Here's how the part is built. I have some questions about the finished solid (model axes, mm). Give positions to 0.01 mm unless a question says otherwise; leave off trailing zeros. Order: outer loops, then holes, each group sorted by start corner. A loop starts at its lowest first (then second) coordinate and runs counter-clockwise, first axis right, second up. Notation, with made-up numbers: (40.5, 53.5) - (98.5, 53.5) arc R15 ccw to (98.5, 69.5) - close; hole circle Ø8 at (41.25, 40). An arc over 180 degrees is marked (long way). One line per question, with ' | ' between items.
from build123d import *

# Parameters (mm, degrees)
F1_R     = 12
F2_DEPTH = 15


with BuildPart() as f2:
    # F1 (on face) → F2 (new body)
    with BuildSketch(Plane.XY):
        with BuildLine():
            ThreePointArc((17.8272945993, -129.4724747228), (30.8870152167, -67.4921341785), (35.2682027622, -4.3025455402))
            add(Edge.make_bspline(
                [(35.2682027622, -4.3025455402), (35.2682027622, -2.8630395725), (34.7940906326, 4.5484558025), (29.9290871814, 17.4019463757), (16.1515405759, 28.168861008), (-0.0978770248, 30.3942939385), (-14.2158344876, 24.4556370199), (-22.8083044544, 13.0367090709), (-23.9004306853, -0.1517972714), (-21.1020014845, -7.483800271), (-18.1865334795, -10.5)],
                knots=[0.1989185015, 0.1989185015, 0.1989185015, 0.1989185015, 0.2248112778, 0.3326230217, 0.4372558817, 0.5386130078, 0.6365884477, 0.7310656976, 0.8219159332, 0.9089958388, 0.9089958388, 0.9089958388, 0.9089958388], degree=3))
            ThreePointArc((-18.1865334795, -10.5), (1.139918362, -43.3697806371), (3.3405694731, -81.4367131981))
            ThreePointArc((3.3405694731, -81.4367131981), (1.1378022248, -105.0250778662), (3.0062398837, -128.6422765143))
            ThreePointArc((3.0062398837, -128.6422765143), (10.0845593286, -134.9880938543), (17.8272945993, -129.4724747228))
        make_face()
        Circle(F1_R, mode=Mode.SUBTRACT)
    extrude(amount=F2_DEPTH)


solid = f2.part
1) Please list where these lines run through material, in increasing order: L1, parallel to Y at x = -4, z = 14; L2, parallel to X at y = 7, z = 11.5; L3, parallel to Y at x = -9, z = 9.
Model answer:
L1: y = -30.5 to -11.31, 11.31 to 28.17 | L2: x = -23.02 to -9.75, 9.75 to 33.43 | L3: y = -21.9 to -7.94, 7.94 to 26.23
2) I want a section at B-B (y = -108.5). List the corners of the cut face in (x, z) for me, plus the area to 3 significant figures.
Model answer:
outline: (1.16, 0) - (23.25, 0) - (23.25, 15) - (1.16, 15) - close | area: 331 mm2
3) Thinking about a two-plate mould opening in Y: for faces 1 (the face through (30.764, -68.371, 7.395)), 2 (the face through (12, -33, 15)), 3 (the face through (-11.99, 0.53, 7.4)), which applies, +Y half, -Y half, draft (parallel to the pull), parting line (faces both ways), or undercut?
Model answer:
face 1: -Y half | face 2: draft | face 3: undercut
4) I want a section at A-A (y = -40.5). List the corners of the cut face in (x, z) for me.
Model answer:
outline: (0.21, 0) - (33.84, 0) - (33.84, 15) - (0.21, 15) - close
5) I'm going to push flat-ended pins straight in: P1, Ø1.5, axis at x = -15.5, z = 9.5, coming from the +Y side; P2, Ø1, axis at y = -25.5, z = 12.5, coming from the +X side; P3, Ø3, axis at x = -4.5, z = 6, coming from the +Y side. Where does each tip first touch, or does it pass through?
Model answer:
P1: stops at y = 22.34 | P2: stops at x = 34.8 | P3: stops at y = 28.44
